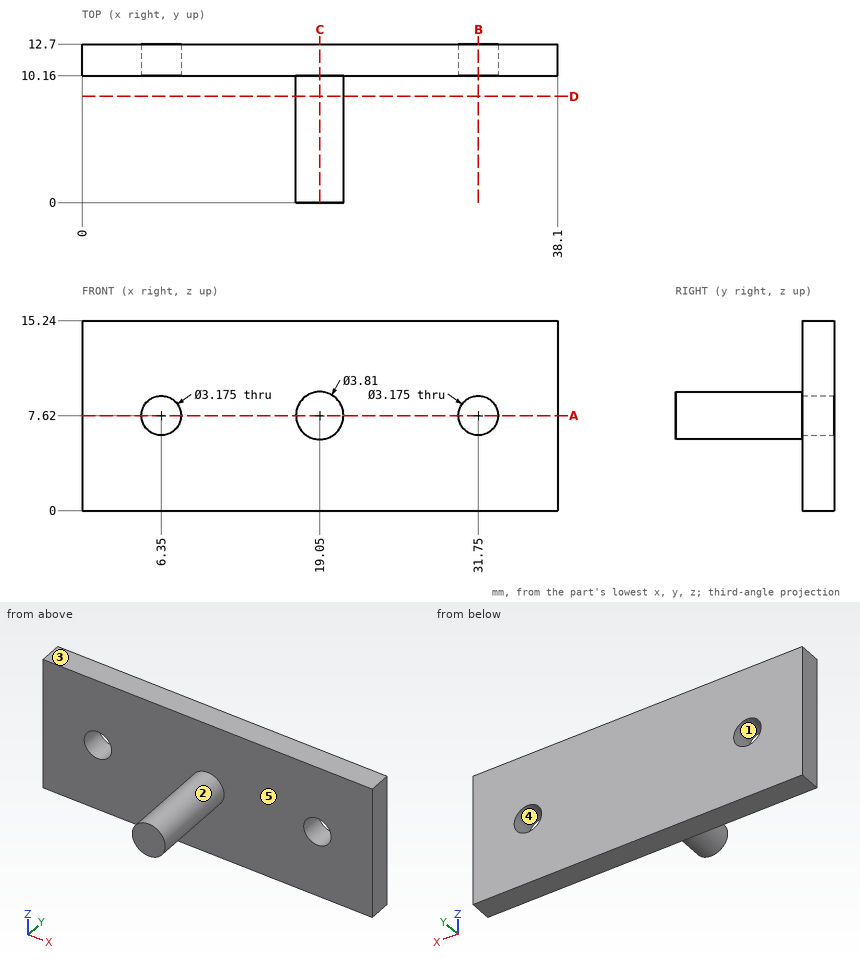
Check sheet for the drawn part. Datum: minimum x, y, z corner. Units: mm. A direction names the side the tool comes from. Round coordinates to 2 decimals unless told otherwise and drop trailing zeros. Order: outer loops, then holes, each group sorted by start corner. A loop starts at its lowest first (then second) coordinate and runs counter-clockwise, first axis right, second up. Notation, with made-up numbers: M -16,35 L 42,35 A8 ccw 42,48 Z; hole C -12,67.25 d4. An arc over 180 degrees is marked long. Write each question's results on one line, items separated by ' | '. Start each with the question number.
1. Cross-section at C-C on x = 19.05. Record the boundary of the cut face in (y, z) (3 decimals), plus the area to 3 significant figures.
2. Material ranges on L1, parallel to X at y = 11.15, z = 7.62; L2, parallel to X at y = 10.25, z = 6.5; L3, parallel to Y at x = 5, z = 3.5, recorded low to high. Write a range as from..to.
3. Cross-section at D-D on y = 8.5. Record the boundary of the cut face in (x, z) (3 decimals), plus the area to 3 significant figures.
4. Set-up check for the marked faces 1 and 2: record each of +Z, -Z, +X, -X, +Y, -Y from which the full face is reachable in a straight line by a thin tool's end or side.
5. Cross-section at B-B on x = 31.75. Record the boundary of the cut face in (y, z).
6. Draft check along Z on the marked faces 3, 4 and 5. Enter one of: pulls with the +Z half, pulls with the -Z half, needs draft (parallel to the pull), parting line crosses it, or undercut.
7. Go/stop test with flat-tipped pins: P1, Ø5, axis at x = 16.5, y = 6.5, coming from the -Z side; P2, Ø8, axis at x = 5.5, z = 10.5, coming from the -Y side. Record where each tip stops, or that it passes through.
8. Cross-section at A-A on z = 7.62. Record the boundary of the cut face in (x, y) (1 decimal), plus the area to 3 significant figures.
Resolved:
1) outline: M 0,5.715 L 10.16,5.715 L 10.16,0 L 12.7,0 L 12.7,15.24 L 10.16,15.24 L 10.16,9.525 L 0,9.525 Z | area: 77.4 mm2
2) L1: 0..4.76, 7.94..30.16, 33.34..38.1 | L2: 0..5.22, 7.48..30.62, 32.88..38.1 | L3: 10.16..12.7
3) outline: C 19.05,7.62 d3.81 | area: 11.4 mm2
4) face 1: +Y, -Y | face 2: -Y
5) outline: M 10.16,0 L 12.7,0 L 12.7,6.03 L 10.16,6.03 Z; M 10.16,9.21 L 12.7,9.21 L 12.7,15.24 L 10.16,15.24 Z
6) face 3: pulls with the +Z half | face 4: undercut | face 5: needs draft
7) P1: z = 5.72 | P2: y = 10.16
8) outline: M 0,10.2 L 4.8,10.2 L 4.8,12.7 L 0,12.7 Z; M 7.9,10.2 L 17.1,10.2 L 17.1,0 L 21,0 L 21,10.2 L 30.2,10.2 L 30.2,12.7 L 7.9,12.7 Z; M 33.3,10.2 L 38.1,10.2 L 38.1,12.7 L 33.3,12.7 Z | area: 119 mm2
